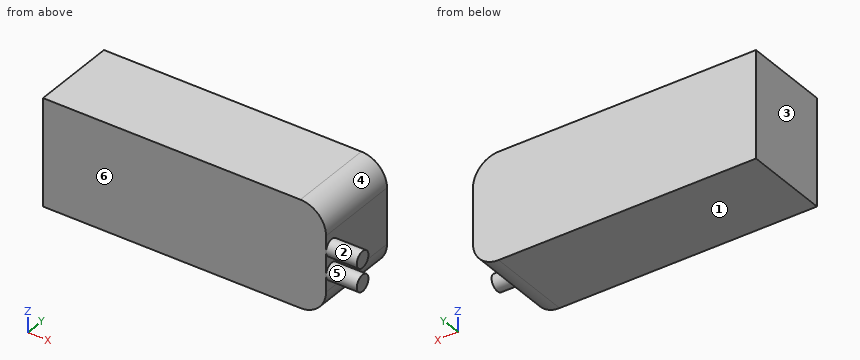
from build123d import *

# Parameters (mm, degrees)
SALIENTE_EXTRUIR1_DEPTH = 42
CROQUIS7_R              = 4
SALIENTE_EXTRUIR2_DEPTH = 15


with BuildPart() as part:
    # Croquis1 → Saliente-Extruir1 (new body)
    with BuildSketch(Plane(origin=(0, 0, 0), x_dir=(1, 0, 0), z_dir=(0, 1, 0))):
        with BuildLine():
            Line((0, 0), (125.5, 0))
            ThreePointArc((125.5, 0), (134.338834765, 3.661165235), (138, 12.5))
            Line((138, 12.5), (138, 39.5))
            ThreePointArc((138, 39.5), (134.338834765, 48.338834765), (125.5, 52))
            Line((125.5, 52), (0, 52))
            Line((0, 52), (0, 0))
        make_face()
    extrude(amount=SALIENTE_EXTRUIR1_DEPTH)

    # Croquis7 → Saliente-Extruir2 (add)
    with BuildSketch(Plane(origin=(138, 0, 0), x_dir=(0, 0, -1), z_dir=(1, 0, 0))):
        with Locations(Location((20.189152703, 4, 0), (0, 0, 270))):
            Circle(CROQUIS7_R)
        with Locations(Location((31.517370161, 4, 0), (0, 0, 270))):
            Circle(CROQUIS7_R)
    extrude(amount=SALIENTE_EXTRUIR2_DEPTH)


solid = part.part
Geometry: final body of the model. Coordinates: model frame, mm. Face numbers are marked on the shaded views. A direction names the side the tool comes from. Give positions to 0.01 mm unless a question says otherwise; leave off trailing zeros. Write each loop counter-clockwise with the first axis right and the second up, starting at its lowest first coordinate (ties: lowest second). Pieces come first, ordered by that corner, then holes. Notation, with made-up numbers: M -18.75,6.25 L 9.25,6.25 A22 cw 9.25,22.25 Z; hole C 22,49.5 d9. An arc over 180 degrees is marked long. Answer in a Markdown table with one row per item. Add a question column.
(1) Reachability of the marked faces 5 and 6 from +Z, -Z, +X, -X, +Y, -Y: full face, straight path, thin tool, end or side. Return the list, or none.
(2) Mould query, pull axis Z, two halves, no side actions, for the marked faces 1, 2, 3 and 4. Classes: +Z half, -Z half, draft (parallel to the pull), parting line (faces both ways), or undercut.
(3) Section C-C on x = 143.5. Return loops of the section in (y, z), and give its area (3 significant figures).
(4) First-contact query: pin 1 (4 mm diameter, centred on y = 19, z = -6.5, fed in from +X); pin 2 (3 mm diameter, centred on y = 28, z = -42.5, fed in from +X); pin 3 (8 mm diameter, centred on y = 13, z = -21, fed in from +X). Flat tips, straight axial feed; report the tip coordinate or a pass-through.
(5) Section A-A on y = 4. Return loops of the section in (x, z).
(6) Ray query, line 1 (X direction, y = 30, z = -33); line 2 (X direction, y = 21.5, z = -45); line 3 (Z direction, x = 129.5, y = 34). Return the intervals inside material, ascending.
(7) Section D-D on y = 26.5. Return loops of the section in (x, z).
(8) Section B-B on z = -33. Return loops of the section in (x, y).
Result set:
| question | item | result |
|---|---|---|
| 1 | face 5 | +X |
| 1 | face 6 | +Z, -Z, +X, -X, -Y |
| 2 | face 1 | -Z half |
| 2 | face 2 | undercut |
| 2 | face 3 | draft |
| 2 | face 4 | +Z half |
| 3 | outline | C 4,-31.52 d8; C 4,-20.19 d8 |
| 3 | area | 101 mm^2 |
| 4 | pin 1 | stops at x = 137.34 |
| 4 | pin 2 | stops at x = 137.91 |
| 4 | pin 3 | stops at x = 138 |
| 5 | outline | M 0,-52 L 125.5,-52 A12.5 ccw 138,-39.5 L 138,-35.52 L 153,-35.52 L 153,-27.52 L 138,-27.52 L 138,-24.19 L 153,-24.19 L 153,-16.19 L 138,-16.19 L 138,-12.5 A12.5 ccw 125.5,0 L 0,0 Z |
| 6 | line 1 | x = 0 to 138 |
| 6 | line 2 | x = 0 to 136.72 |
| 6 | line 3 | z = -51.34 to -0.66 |
| 7 | outline | M 0,-52 L 125.5,-52 A12.5 ccw 138,-39.5 L 138,-12.5 A12.5 ccw 125.5,0 L 0,0 Z |
| 8 | outline | M 0,0 L 138,0 L 138,0.28 L 153,0.28 L 153,7.72 L 138,7.72 L 138,42 L 0,42 Z |
